from build123d import *

# Parameters (mm, degrees)
SKETCH1_R           = 2
SKETCH1_R_2         = 11
SKETCH1_R_3         = 1.5
BOSS_EXTRUDE1_DEPTH = 5
FILLET1_R           = 2
FILLET2_R           = 15


with BuildPart() as part:
    # Sketch1 → Boss-Extrude1 (new body)
    with BuildSketch(Plane.XY):
        Polygon((0, 0), (6.5, 0), (6.5, -35), (79.5, -35), (79.5, 0), (86, 0), (86, 12.6), (0, 12.6), align=None)
        with Locations((69.5, 7.6)):
            Circle(SKETCH1_R, mode=Mode.SUBTRACT)
        with Locations((16.5, 7.6)):
            Circle(SKETCH1_R, mode=Mode.SUBTRACT)
        with Locations((43, -14)):
            Circle(SKETCH1_R_2, mode=Mode.SUBTRACT)
        with Locations((27.5, -29.5)):
            Circle(SKETCH1_R_3, mode=Mode.SUBTRACT)
        with Locations((58.5, -29.5)):
            Circle(SKETCH1_R_3, mode=Mode.SUBTRACT)
        with Locations((27.5, 1.5)):
            Circle(SKETCH1_R_3, mode=Mode.SUBTRACT)
        with Locations((58.5, 1.5)):
            Circle(SKETCH1_R_3, mode=Mode.SUBTRACT)
        with BuildLine():
            Line((13.745004537, -11.1), (19.254995463, -11.1))
            ThreePointArc((19.254995463, -11.1), (16.5, -18), (13.745004537, -11.1))
        make_face(mode=Mode.SUBTRACT)
        with BuildLine():
            Line((66.745004537, -11.1), (72.254995463, -11.1))
            ThreePointArc((72.254995463, -11.1), (69.5, -18), (66.745004537, -11.1))
        make_face(mode=Mode.SUBTRACT)
    extrude(amount=BOSS_EXTRUDE1_DEPTH)

    # Fillet1
    fillet1_edges = [part.edges().sort_by_distance(p)[0] for p in [
        (0, 12.6, 2.5),
        (86, 12.6, 2.5),
        (86, 0, 2.5),
        (79.5, 0, 2.5),
        (6.5, 0, 2.5),
        (0, 0, 2.5),
    ]]
    fillet(fillet1_edges, radius=FILLET1_R)

    # Fillet2
    fillet2_edges = [part.edges().sort_by_distance(p)[0] for p in [
        (79.5, -35, 2.5),
        (6.5, -35, 2.5),
    ]]
    fillet(fillet2_edges, radius=FILLET2_R)


solid = part.part
Here's how the part is built. I have some questions about the finished solid (model axes, mm). A direction names the side the tool comes from. Coordinates: 2 decimals unless noted, no trailing zeros. Order: outer loops, then holes, each group sorted by start corner. A loop starts at its lowest first (then second) coordinate and runs counter-clockwise, first axis right, second up. Notation, with made-up numbers: M 69,52 L 104,52 A18 cw 104,70 Z; hole C 67,75.5 d3. An arc over 180 degrees is marked long. Answer as CSV lines item,"result". Start each with the question number.
1. I want a section at D-D, the plane y = 7.6. Write out the boundary of the cut face in (x, z), and give its area (3 significant figures).
2. I need wall thicknesses on line 1 (Y direction, x = 27.5, z = 1.1); line 2 (X direction, y = 0.5, z = 3.4); line 3 (Y direction, x = 16.5, z = 3.9). Which ranges of each line are inside material? Lowest first, please. Write a range as [from, to].
3. We'd pull the mould along X, two halves only. Please class faces 1 (the flat face through (6.5, -11, 2)), 2 (the cylindrical face through (14.502, 7.688, 2.465)), 3 (the flat face through (42, 0, 5)): released by +X, released by -X, zero draft, split by the parting line, or undercut.
4. For pin 1 (1.2 mm diameter, centred on x = 82.5, z = 2, fed in from -Y); pin 2 (2.5 mm diameter, centred on y = -12, z = 2.5, fed in from +X); pin 3 (1.5 mm diameter, centred on y = -10.5, z = 1.5, fed in from -X); pin 4 (2.5 mm diameter, centred on x = 69.5, y = 7.6, fed in from +Z), each with a flat end and sliding along its axis, tell me the tip position at first contact or that it passes through.
5. On a 3-axis mill with a long thin cutter (end or side, diameter ignored), from which of +Z, -Z, +X, -X, +Y, -Y can I reach the whole of each face in a straight line? I mean faces 4 (the cylindrical face through (5.9, -0.57, 2.54)), 5 (the flat face through (79.5, -11, 2)). Say none if no direction works.
6. I want a section at C-C, the plane z = 2.1. Count the separate pieces of the cut face and the enclosed holes in it, and give its area (3 significant figures).
7. I want a section at B-B, the plane x = 43. Write out the boundary of the cut face in (y, z).
8. I want a section at A-A, the plane y = -14. Write out the boundary of the cut face in (x, z).
Recorded:
1,outline,"M 0,0 L 14.5,0 L 14.5,5 L 0,5 Z; M 18.5,0 L 67.5,0 L 67.5,5 L 18.5,5 Z; M 71.5,0 L 86,0 L 86,5 L 71.5,5 Z"
1,area,"390 mm2"
2,line 1,"y = [-35, -31], [-28, 0], [3, 12.6]"
2,line 2,"x = [0.68, 26.38], [28.62, 57.38], [59.62, 85.32]"
2,line 3,"y = [-34.14, -18], [-11.1, 5.6], [9.6, 12.6]"
3,face 1,"released by -X"
3,face 2,"undercut"
3,face 3,"zero draft"
4,pin 1,"stops at y = 0"
4,pin 2,"stops at x = 79.5"
4,pin 3,"stops at x = 6.5"
4,pin 4,"passes through"
5,face 4,"+Z, -Z, -X, -Y"
5,face 5,"+Z, -Z, +X, -Y"
6,separate pieces,"1"
6,enclosed holes,"9"
6,area,"3,010 mm2"
7,outline,"M -35,0 L -25,0 L -25,5 L -35,5 Z; M -3,0 L 12.6,0 L 12.6,5 L -3,5 Z"
8,outline,"M 6.5,0 L 12.5,0 L 12.5,5 L 6.5,5 Z; M 20.5,0 L 32,0 L 32,5 L 20.5,5 Z; M 54,0 L 65.5,0 L 65.5,5 L 54,5 Z; M 73.5,0 L 79.5,0 L 79.5,5 L 73.5,5 Z"
